The listing builds one solid part. Answer for the finished solid, in the listing's coordinates (mm). A direction names the side the tool comes from. Give positions to 0.01 mm unless a question says otherwise; leave off trailing zeros. Order: outer loops, then holes, each group sorted by start corner. A loop starts at its lowest first (then second) coordinate and runs counter-clockwise, first axis right, second up. Notation, with made-up numbers: (35.25, 61) - (64.25, 61) arc R18 ccw to (64.25, 77) - close; hole circle Ø9 at (-39.5, -17). An arc over 180 degrees is marked (long way). Answer as a JSON object with one key per item and string values. Group by question number.
Q1. Consider line 1 (Y direction, x = 86, z = 1.3); line 2 (Y direction, x = 94, z = 1.7); line 3 (Y direction, x = 77, z = 1). Determine where each line is inside the solid, lowest interval first.
Q2. Given pin 1 (5.5 mm diameter, centred on x = 118.83, y = 4.6, fed in from +Z); pin 2 (1.5 mm diameter, centred on y = 2.5, z = 1.5, fed in from +X); pin 3 (1 mm diameter, centred on x = 92.5, y = -11.5, fed in from +Z), each flat-ended and moving along its own axis, determine where each tip first touches the part or whether it passes through.
Q3. The mould has two halves that part along X. Classify faces 4 (the face through (115.27, -13.13, 2.03)), 5 (the face through (80, -7, 2)), 6 (the face through (75, 2, 0)): released by +X, released by -X, zero draft, split by the parting line, or undercut.
Q4. A cutting plane is placed at A-A, the plane x = 23.95. Give the vertices of the cut face in (y, z), and give its area (3 significant figures).
Q5. A cutting plane is placed at B-B, the plane z = 1.9. Give the vertices of the cut face in (x, y), and give its area (3 significant figures).
Q6. For faces 1 (the face through (121.86, -4.53, 1.97)), 2 (the face through (90.927, -7.483, 2.028)), 3 (the face through (39, 0, 2)), determine the directions among +Z, -Z, +X, -X, +Y, -Y from which every point of the face is accessible in a straight line to the end or side of a thin tool.
Q7. A cutting plane is placed at C-C, the plane y = -3. Give the vertices of the cut face in (x, z), and give its area (3 significant figures).
Q8. A cutting plane is placed at D-D, the plane y = 6.25. Give the vertices of the cut face in (x, z).
from build123d import *

# Parameters (mm, degrees)
PAD_DEPTH    = 4
SKETCH001_R  = 3.15
POCKET_DEPTH = 5


with BuildPart() as part:
    # Sketch → Pad (new body)
    with BuildSketch(Plane.XY):
        Polygon((0, 9.2), (0, 0), (80, 0), (80, -13.7), (119.781694, -17.873343), (124, 9.2), align=None)
    extrude(amount=PAD_DEPTH)

    # Sketch001 (on DatumPlane) → Pocket (cut)
    with BuildSketch(Plane.XY.offset(4)):
        with Locations((23.95, 4.6)):
            Circle(SKETCH001_R)
        with Locations((118.83, 4.6)):
            Circle(SKETCH001_R)
        Polygon((84, 0), (118.83, 0), (115.67, -8.7), (84, -4.07), align=None)
        Polygon((84, -6.47), (98.050642, -8.524135), (97.44308, -12.679959), (83.392439, -10.625824), align=None)
        Polygon((101.52, -9.03), (115.570642, -11.084135), (114.96308, -15.239959), (100.912439, -13.185824), align=None)
    extrude(amount=-POCKET_DEPTH, mode=Mode.SUBTRACT)


solid = part.part
Reply:
{
 "1": {"line 1": "y = -14.33 to -11.01, -6.76 to -4.36, 0 to 9.2", "line 2": "y = -15.17 to -12.18, -7.93 to -5.53, 0 to 9.2", "line 3": "y = 0 to 9.2"},
 "2": {"pin 1": "passes through", "pin 2": "stops at x = 123.07", "pin 3": "stops at z = 4"},
 "3": {"face 4": "undercut", "face 5": "released by -X", "face 6": "zero draft"},
 "4": {"outline": "(0, 0) - (1.45, 0) - (1.45, 4) - (0, 4) - close; (7.75, 0) - (9.2, 0) - (9.2, 4) - (7.75, 4) - close", "area": "11.6 mm^2"},
 "5": {"outline": "(0, 0) - (80, 0) - (80, -13.7) - (119.78, -17.87) - (124, 9.2) - (0, 9.2) - close; hole circle Ø6.3 at (23.95, 4.6); hole (83.39, -10.63) - (97.44, -12.68) - (98.05, -8.52) - (84, -6.47) - close; hole (84, -4.07) - (115.67, -8.7) - (118.83, 0) - (84, 0) - close; hole (100.91, -13.19) - (114.96, -15.24) - (115.57, -11.08) - (101.52, -9.03) - close; hole circle Ø6.3 at (118.83, 4.6)", "area": "1,390 mm^2"},
 "6": {"face 1": "+Z, -Z, +X, -Y", "face 2": "+Z, -Z", "face 3": "+Z, -Z, -X, -Y"},
 "7": {"outline": "(80, 0) - (84, 0) - (84, 4) - (80, 4) - close; (117.74, 0) - (122.1, 0) - (122.1, 4) - (117.74, 4) - close", "area": "33.4 mm^2"},
 "8": {"outline": "(0, 0) - (21.27, 0) - (21.27, 4) - (0, 4) - close; (26.63, 0) - (116.15, 0) - (116.15, 4) - (26.63, 4) - close; (121.51, 0) - (123.54, 0) - (123.54, 4) - (121.51, 4) - close"}
}
